Part model, mm, in its own coordinate system. Face numbers are marked on the shaded views. A direction names the side the tool comes from. Give positions to 0.01 mm unless a question says otherwise; leave off trailing zeros. Order: outer loops, then holes, each group sorted by start corner. A loop starts at its lowest first (then second) coordinate and runs counter-clockwise, first axis right, second up. Notation, with made-up numbers: M 21.25,-13 L 60.25,-13 A28 cw 60.25,25 Z; hole C 32.5,51.5 d10. An arc over 180 degrees is marked long. Return JSON: item names as keys, results as strings.
from build123d import *

# Parameters (mm, degrees)
SKETCH1_R               = 5
BOSS_EXTRUDE1_DEPTH     = 16
SKETCH2_W               = 8
SKETCH2_H               = 22
CUT_EXTRUDE1_DEPTH      = 8
CUT_EXTRUDE1_DEPTH_BACK = 8
FILLET1_R               = 1
CUT_EXTRUDE2_DEPTH      = 17
FILLET2_R               = 5


with BuildPart() as part:
    # Sketch1 → Boss-Extrude1 (new body)
    with BuildSketch(Plane(origin=(0, 0, 0), x_dir=(0, 0, -1), z_dir=(1, 0, 0))):
        with BuildLine():
            Line((0, 7), (50, 7))
            ThreePointArc((50, 7), (57, 0), (50, -7))
            Line((50, -7), (0, -7))
            ThreePointArc((0, -7), (-7, 0), (0, 7))
        make_face()
        Circle(SKETCH1_R, mode=Mode.SUBTRACT)
        with Locations((50, 0)):
            Circle(SKETCH1_R, mode=Mode.SUBTRACT)
    extrude(amount=BOSS_EXTRUDE1_DEPTH)

    # Sketch2 → Cut-Extrude1 (cut, two sides)
    with BuildSketch(Plane(origin=(0, 0, 0), x_dir=(1, 0, 0), z_dir=(0, 1, 0))) as cut_extrude1_sk:
        with Locations((8, 4)):
            Rectangle(SKETCH2_W, SKETCH2_H)
        with Locations((8, 46)):
            Rectangle(SKETCH2_W, SKETCH2_H)
    extrude(amount=CUT_EXTRUDE1_DEPTH, mode=Mode.SUBTRACT)
    extrude(cut_extrude1_sk.sketch, amount=-CUT_EXTRUDE1_DEPTH_BACK, mode=Mode.SUBTRACT)

    # Fillet1
    fillet1_edges = [part.edges().sort_by_distance(p)[0] for p in [
        (12, 0, -15),
        (4, 0, -15),
        (4, 0, -35),
        (12, 0, -35),
    ]]
    fillet(fillet1_edges, radius=FILLET1_R)

    # Sketch3 → Cut-Extrude2 (cut, through all)
    with BuildSketch(Plane(origin=(16, 0, 0), x_dir=(0, 0, -1), z_dir=(1, 0, 0))):
        with BuildLine():
            Line((13.884919825, -4), (36.115080175, -4))
            ThreePointArc((36.115080175, -4), (37.449748085, -4.181425359), (38.687558952, -4.712535371))
            Line((38.687558952, -4.712535371), (42.5, -7))
            Line((42.5, -7), (7.5, -7))
            Line((7.5, -7), (11.312441048, -4.712535371))
            ThreePointArc((11.312441048, -4.712535371), (12.550251915, -4.181425359), (13.884919825, -4))
        make_face()
        with BuildLine():
            Line((11.312441048, 4.712535371), (7.5, 7))
            Line((7.5, 7), (42.5, 7))
            Line((42.5, 7), (38.687558952, 4.712535371))
            ThreePointArc((38.687558952, 4.712535371), (37.449748085, 4.181425359), (36.115080175, 4))
            Line((36.115080175, 4), (13.884919825, 4))
            ThreePointArc((13.884919825, 4), (12.550251915, 4.181425359), (11.312441048, 4.712535371))
        make_face()
    extrude(amount=-CUT_EXTRUDE2_DEPTH, mode=Mode.SUBTRACT)

    # Fillet2
    fillet2_edges = [part.edges().sort_by_distance(p)[0] for p in [
        (2, -7, -7.5),
        (14, -7, -7.5),
        (14, -7, -42.5),
        (2, -7, -42.5),
        (2, 7, -42.5),
        (14, 7, -42.5),
        (2, 7, -7.5),
        (14, 7, -7.5),
    ]]
    fillet(fillet2_edges, radius=FILLET2_R)


solid = part.part
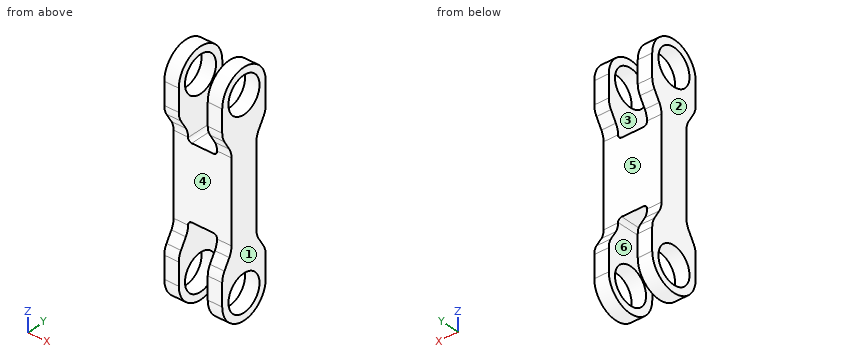
Q1. Band-saw the part on B-B (z = -39.5). Give the cut face in (x, y), then the cut area to 3 significant figures.
Established:
{"outline": "M 0,-5.2 L 4,-5.2 L 4,5.2 L 0,5.2 Z; M 12,-5.2 L 16,-5.2 L 16,5.2 L 12,5.2 Z", "area": "83.2 mm²"}
Q2. Probe line 1 along Y through (x, z) = (13.9, -50); line 2 along Z through (x, y) = (14.75, 4.5); line 3 along Z through (x, y) = (1.65, 0). List the from-to ranges inside material, lowest first.
Established:
{"line 1": "y = -7 to -5, 5 to 7", "line 2": "z = -55.36 to -52.18, -47.82 to -38.29, -11.71 to -2.18, 2.18 to 5.36", "line 3": "z = -57 to -55, -45 to -5, 5 to 7"}
Q3. Band-saw the part on C-C (y = 0). Give the number of separate pieces and of enclosed holes in the cut face, then the cut area to 3 significant figures.
Established:
{"separate pieces": "5", "enclosed holes": "0", "area": "513 mm²"}
Q4. Band-saw the part on A-A (x = 13.25). Give the cut face in (y, z).
Established:
{"outline": "M -7,-50 A7 ccw 7,-50 L 7,-43.88 A5 ccw 6.29,-41.31 L 4.71,-38.69 A5 cw 4,-36.12 L 4,-13.88 A5 cw 4.71,-11.31 L 6.29,-8.69 A5 ccw 7,-6.12 L 7,0 A7 ccw -7,0 L -7,-6.12 A5 ccw -6.29,-8.69 L -4.71,-11.31 A5 cw -4,-13.88 L -4,-36.12 A5 cw -4.71,-38.69 L -6.29,-41.31 A5 ccw -7,-43.88 Z; hole C 0,-50 d10; hole C 0,0 d10"}
Q5. Two-plate mould, pull along X, no slides. Class the marked faces 1, 2 and 3: +X half, -X half, draft (parallel to the pull), parting line (faces both ways), or undercut.
Established:
{"face 1": "+X half", "face 2": "-X half", "face 3": "undercut"}
Q6. 3-axis set-ups, long thin cutter, end or side, ignore diameter. For the marked faces 4, 5 and 6: which of +Z, -Z, +X, -X, +Y, -Y reach the whole face in a straight line?
Established:
{"face 4": "+X, -X, -Y", "face 5": "+X, -X, +Y", "face 6": "-Z, +Y, -Y"}
Q7. Pin check, flat tips, straight feed: pin 1 (1.8 mm diameter, centred on x = 8, y = -0.5, fed in from -Z); pin 2 (4 mm diameter, centred on x = 14.5, y = 5, fed in from +Z); pin 3 (8 mm diameter, centred on x = 5, z = -27.5, fed in from -Y). Stop position of each tip, or through.
Established:
{"pin 1": "stops at z = -35", "pin 2": "stops at z = 6.32", "pin 3": "stops at y = -4"}
Q8. Band-saw the part on D-D (z = -12). Give the cut face in (x, y), then the cut area to 3 significant figures.
Established:
{"outline": "M 0,-4.37 L 4,-4.37 L 4,4.37 L 0,4.37 Z; M 12,-4.37 L 16,-4.37 L 16,4.37 L 12,4.37 Z", "area": "69.9 mm²"}
